For this review, take the finished solid that the model builds, in its own axes (mm). A direction names the side the tool comes from. Round coordinates to 2 decimals unless told otherwise and drop trailing zeros. Write each loop counter-clockwise with the first axis right and the second up, starting at its lowest first coordinate (ties: lowest second). Pieces come first, ordered by that corner, then holes. Notation, with made-up numbers: (-33.5, 25) -> (0.5, 25) arc R3 cw to (0.5, 30) -> close; hole circle Ø6 at (77, 10.5). An arc over 180 degrees is marked (long way). Write each question's results on one line, items separated by ' | '. Start each with the question number.
Item 1: To check wall thickness, follow line 1 along Z through (x, y) = (-8, -9.5); line 2 along Y through (x, z) = (-10.5, 36.5); line 3 along Z through (x, y) = (-7.5, 17.15). State the ranges of each line that lie inside material, in increasing order.
Item 2: Tool access review of faces 5 (the flat face through (-6, -15, 32)), 6 (the cylindrical face through (-5.916, 13.423, 2.981)): name each direction out of +Z, -Z, +X, -X, +Y, -Y from which nothing blocks a thin tool from reaching the whole face with its end or side.
Item 3: Add section B-B (x = -5). State the section outline as (y, z) points.
Item 4: Add section C-C (y = -17.15). State the section outline as (x, z) points, plus the area to 3 significant figures.
Item 5: Clearance check with flat-ended pins moving along their axes: pin 1 (1 mm diameter, centred on x = -9.5, y = -20, fed in from +Z); pin 2 (7 mm diameter, centred on x = -6, z = 38.5, fed in from +Y); pin 3 (1 mm diameter, centred on x = -10.5, y = -17.5, fed in from +Z). State where each tip first meets the part, or that it passes through.
Item 6: The part is to be moulded in two halves that separate along Y. For faces 1 (the flat face through (-6, -25, 0)), 2 (the flat face through (-3, 0, 44.5)), 3 (the cylindrical face through (-6.084, -18.724, 0.496)), 4 (the flat face through (-6, 15, 31)), say which applies: +Y half, -Y half, draft (parallel to the pull), parting line (faces both ways), or undercut.
Item 7: Add section D-D (x = -1). State the section outline as (y, z) points, plus the area to 3 significant figures.
Item 8: Add section A-A (y = 0). State the section outline as (x, z) points, plus the area to 3 significant figures.
from build123d import *

# Parameters (mm, degrees)
F1_DEPTH = 12
F3_D     = 3.3
F4_R     = 3
F5_DEPTH = 30
F6_R     = 6


with BuildPart() as f1:
    # F0 (on Right) → F1 (new body)
    with BuildSketch(Plane.YZ):
        Polygon((15, 44.5), (0, 44.5), (-15, 44.5), (-15, 18.5), (-25, 2.5), (-25, -2.5), (-15, -18.5), (0, -18.5), (15, -18.5), (25, -2.5), (25, 2.5), (15, 18.5), align=None)
        with BuildLine():
            ThreePointArc((0, 13.75), (13.75, 0), (0, -13.75))
            ThreePointArc((0, -13.75), (-13.75, 0), (0, 13.75))
        make_face(mode=Mode.SUBTRACT)
    extrude(amount=-F1_DEPTH)

    # F3 (through all)
    with Locations(Plane.YZ):
        with Locations((-17.15, 0), (17.15, 0)):
            Hole(F3_D / 2)

    # F4 (on face) → F5 (cut, through all)
    with BuildSketch(Plane.XZ.offset(15)):
        with Locations((-6, 38.5)):
            Circle(F4_R)
    extrude(amount=-F5_DEPTH, mode=Mode.SUBTRACT)

    # F6
    f6_edges = [f1.edges().sort_by_distance(p)[0] for p in [
        (-12, 0, 44.5),
    ]]
    fillet(f6_edges, radius=F6_R)


solid = f1.part
Responses:
1) line 1: z = -18.5 to -9.94, 9.94 to 36.26, 40.74 to 44.16 | line 2: y = -15 to 15 | line 3: z = -15.06 to -1.65, 1.65 to 15.06
2) face 5: +Z, +X, -X, -Y | face 6: +X, -X
3) outline: (-25, -2.5) -> (-15, -18.5) -> (15, -18.5) -> (25, -2.5) -> (25, 2.5) -> (15, 18.5) -> (15, 35.67) -> (-15, 35.67) -> (-15, 18.5) -> (-25, 2.5) -> close; (-15, 41.33) -> (15, 41.33) -> (15, 44.5) -> (-15, 44.5) -> close; hole circle Ø3.3 at (-17.15, 0); hole circle Ø27.5 at (0, 0); hole circle Ø3.3 at (17.15, 0)
4) outline: (-12, -15.06) -> (0, -15.06) -> (0, -1.65) -> (-12, -1.65) -> close; (-12, 1.65) -> (0, 1.65) -> (0, 15.06) -> (-12, 15.06) -> close | area: 322 mm^2
5) pin 1: stops at z = 11.3 | pin 2: stops at y = 15 | pin 3: stops at z = 15.3
6) face 1: -Y half | face 2: draft | face 3: undercut | face 4: +Y half
7) outline: (-25, -2.5) -> (-15, -18.5) -> (15, -18.5) -> (25, -2.5) -> (25, 2.5) -> (15, 18.5) -> (15, 44.5) -> (-15, 44.5) -> (-15, 18.5) -> (-25, 2.5) -> close; hole circle Ø3.3 at (-17.15, 0); hole circle Ø27.5 at (0, 0); hole circle Ø3.3 at (17.15, 0) | area: 1,700 mm^2
8) outline: (-12, -18.5) -> (0, -18.5) -> (0, -13.75) -> (-12, -13.75) -> close; (-12, 13.75) -> (0, 13.75) -> (0, 44.5) -> (-6, 44.5) arc R6 ccw to (-12, 38.5) -> close; hole circle Ø6 at (-6, 38.5) | area: 390 mm^2
